The listing builds one solid part. Answer for the finished solid, in the listing's coordinates (mm). A direction names the side the tool comes from. Round coordinates to 2 decimals unless told otherwise and drop trailing zeros. Write each loop counter-clockwise with the first axis right and the second up, starting at its lowest first coordinate (ties: lowest second). Pieces come first, ordered by that corner, then holes. Notation, with made-up numbers: M -4.75,25.25 L 35.25,25.25 A28 cw 35.25,57.25 Z; hole C 39.25,19.5 d5. An arc over 180 degrees is marked long. One line per item, written item: value. Start each with the question number.
(1) Section B-B (x = 28.5) is taken. Determine the outline of the cut face in (y, z).
(2) Section C-C (y = 1.5) is taken. Determine the outline of the cut face in (x, z), plus the area to 3 significant figures.
(3) Consider probe 1 along X at (y, z) = (-1, 3.25); probe 2 along X at (y, z) = (-1.5, -1.5); probe 3 along Z at (x, y) = (5.5, -1.5). Determine where each line is inside the solid, lowest interval first.
(4) Section D-D (y = 3.5) is taken. Determine the outline of the cut face in (x, z).
(5) For faces 5 (the flat face through (24, 2, -1)), 6 (the flat face through (-5, 1, -2)), 7 (the flat face through (-1.35, 0, 0)), determine the directions among +Z, -Z, +X, -X, +Y, -Y from which every point of the face is accessible in a straight line to the end or side of a thin tool.
(6) For a pull along Y with two mould halves and no side action, classify faces 1 (the flat face through (-3.2, 0.99, 1.74)), 2 (the flat face through (40, 0, 0)), 3 (the cylindrical face through (31.888, 1.917, 0.604)), 4 (the flat face through (-3.201, 1.014, -1.724)) as released by +Y, released by -Y, zero draft, split by the parting line, or undercut.
(7) Given P1, Ø4, axis at x = 7.5, y = 2.5, coming from the -Z side; P2, Ø1.2, axis at y = 0, z = -1, coming from the -X side; P3, Ø1, axis at x = 30.5, y = -3, coming from the -Z side; P4, Ø1, axis at x = 8.5, y = 0, coming from the +Z side, each flat-ended and moving along its own axis, determine where each tip first touches the part or whether it passes through.
(8) Section A-A (z = 0) is taken. Determine the outline of the cut face in (x, y), plus the area to 3 significant figures.
```python
from build123d import *

# Parameters (mm, degrees)
SCHNITT_LINEAR_AUSTRAGEN1_DEPTH = 3.65
SKIZZE3_R                       = 2.5
AUFSATZ_LINEAR_AUSTRAGEN1_DEPTH = 24


with BuildPart() as part:
    # Skizze1 → Basis-Rotation (revolve)
    with BuildSketch(Plane.XY):
        Polygon((40, 0), (40, 2.0095), (0, 2.0095), (0, 4.25), (-5, 4.25), (-5, 0), align=None)
    revolve(axis=Axis((0, 0, 0), (1, 0, 0)))

    # Skizze2 → Schnitt-Linear austragen1 (cut)
    with BuildSketch(Plane.ZY.offset(5)):
        Polygon((2.309401077, 0), (1.154700538, 2), (-1.154700538, 2), (-2.309401077, 0), (-1.154700538, -2), (1.154700538, -2), align=None)
    extrude(amount=-SCHNITT_LINEAR_AUSTRAGEN1_DEPTH, mode=Mode.SUBTRACT)

    # Skizze3 → Aufsatz-Linear austragen1 (add)
    with BuildSketch(Plane(origin=(0, 0, 0), x_dir=(0, 0, -1), z_dir=(1, 0, 0))):
        Circle(SKIZZE3_R)
    extrude(amount=AUFSATZ_LINEAR_AUSTRAGEN1_DEPTH)


solid = part.part
```
Recorded:
1. outline: C 0,0 d4.02
2. outline: M -5,-3.98 L 0,-3.98 L 0,-2 L 24,-2 L 24,-1.34 L 40,-1.34 L 40,1.34 L 24,1.34 L 24,2 L 0,2 L 0,3.98 L -5,3.98 L -5,1.44 L -1.35,1.44 L -1.35,-1.44 L -5,-1.44 Z
2. area: 168 mm2
3. probe 1: x = -5 to 0
3. probe 2: x = -5 to 24
3. probe 3: z = -2 to 2
4. outline: M -5,-2.41 L 0,-2.41 L 0,2.41 L -5,2.41 Z
5. face 5: +X
5. face 6: +Z, -Z, -X, +Y, -Y
5. face 7: -X
6. face 1: undercut
6. face 2: zero draft
6. face 3: split by the parting line
6. face 4: undercut
7. P1: stops at z = -2.45
7. P2: stops at x = -1.35
7. P3: passes through
7. P4: stops at z = 2.5
8. outline: M -5,-4.25 L 0,-4.25 L 0,-2.5 L 24,-2.5 L 24,-2.01 L 40,-2.01 L 40,2.01 L 24,2.01 L 24,2.5 L 0,2.5 L 0,4.25 L -5,4.25 L -5,2 L -1.35,2 L -1.35,-2 L -5,-2 Z
8. area: 212 mm2
